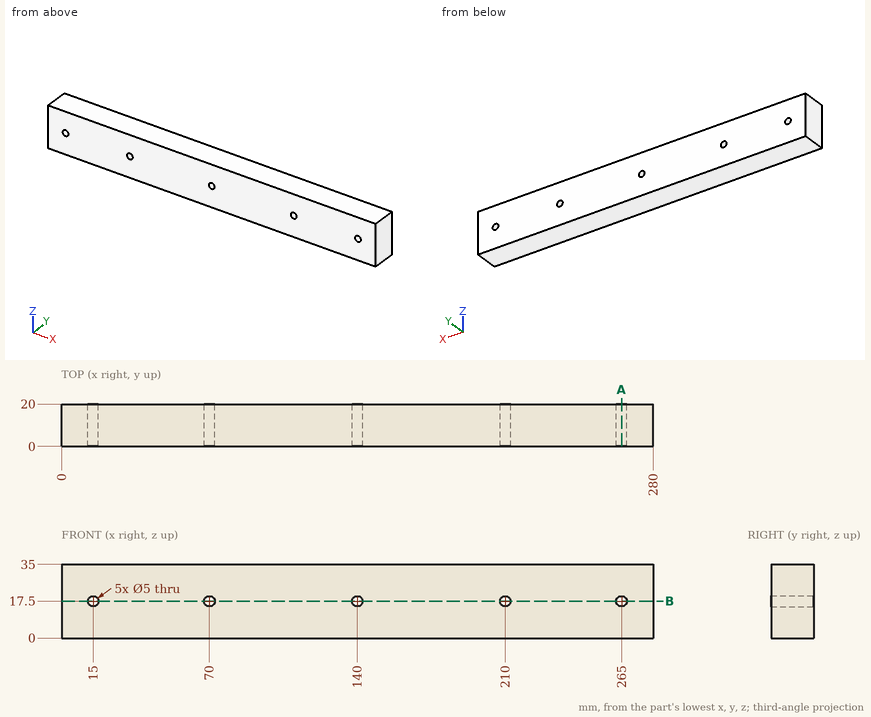
Could you check a few things on this drawing? It's one solid part, dimensions in mm from its lowest x, y, z. Coordinates: 2 decimals unless noted, no trailing zeros. Loops run counter-clockwise (first coordinate to the right, second up) from the corner with the lowest first, then second, coordinate; pieces in that order, holes last. Notation, with made-up numbers: (64.25, 30.5) - (122.25, 30.5) arc R19 ccw to (122.25, 42.5) - close; hole circle Ø6 at (73, 78). An arc over 180 degrees is marked (long way). Return JSON: item names as keys, results as strings. Group by question number.
Item 1: If we section it at A-A on x = 265: Write out the boundary of the cut face in (y, z).
Item 2: If we section it at B-B on z = 17.5: Write out the boundary of the cut face in (x, y).
Item 3: I need wall thicknesses on line 1 (X direction, y = 16, z = 17.5); line 2 (Z direction, x = 140, y = 15); line 3 (X direction, y = 16.25, z = 16.5). Which ranges of each line are inside material? Lowest first, please. Write a range as from..to.
Calculated:
{
 "1": {"outline": "(0, 0) - (20, 0) - (20, 15) - (0, 15) - close; (0, 20) - (20, 20) - (20, 35) - (0, 35) - close"},
 "2": {"outline": "(0, 0) - (12.5, 0) - (12.5, 20) - (0, 20) - close; (17.5, 0) - (67.5, 0) - (67.5, 20) - (17.5, 20) - close; (72.5, 0) - (137.5, 0) - (137.5, 20) - (72.5, 20) - close; (142.5, 0) - (207.5, 0) - (207.5, 20) - (142.5, 20) - close; (212.5, 0) - (262.5, 0) - (262.5, 20) - (212.5, 20) - close; (267.5, 0) - (280, 0) - (280, 20) - (267.5, 20) - close"},
 "3": {"line 1": "x = 0..12.5, 17.5..67.5, 72.5..137.5, 142.5..207.5, 212.5..262.5, 267.5..280", "line 2": "z = 0..15, 20..35", "line 3": "x = 0..12.71, 17.29..67.71, 72.29..137.71, 142.29..207.71, 212.29..262.71, 267.29..280"}
}
